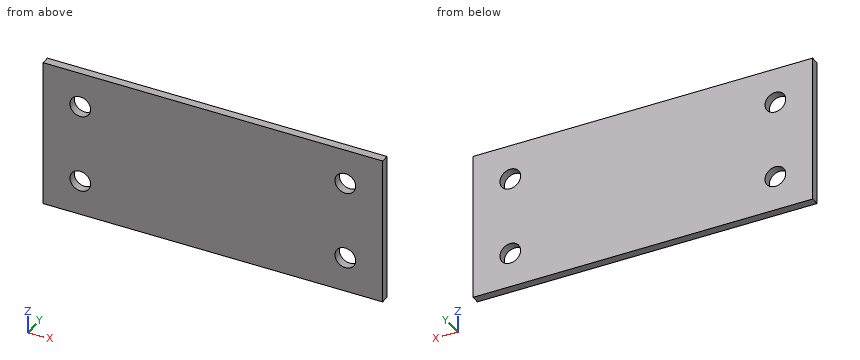
Autodesk Inventor part; units mm, degrees
ref_plane "YZ Plane" through (0, 0, 0) normal (1, 0, 0) x (0, 1, 0)
ref_plane "XZ Plane" through (0, 0, 0) normal (0, 1, 0) x (-1, 0, 0)
ref_plane "XY Plane" through (0, 0, 0) normal (0, 0, 1) x (1, 0, 0)
sketch "Sketch1" plane through (0, 0, 0) normal (0, 1, 0) x (-1, 0, 0)
  line L0 (0, -40.005) -> (0, 40.005)
  line L1 (91.1225, 0) -> (-91.1225, 0)
  line L2 (65.0875, -28.575) -> (-65.0875, -28.575)
  line L3 (-65.0875, -28.575) -> (-65.0875, 28.575)
  line L4 (-65.0875, 28.575) -> (65.0875, 28.575)
  line L5 (65.0875, 28.575) -> (65.0875, -28.575)
  circle A0 centre (50.8, -15.0812) radius 3.9688
  circle A1 centre (50.8, 15.0812) radius 3.9688
  circle A2 centre (-50.8, -15.0812) radius 3.9688
  circle A3 centre (-50.8, 15.0812) radius 3.9688
  point P0 (0, 0)
  dimension "d0" = 130.175
  dimension "d1" = 57.15
  dimension "d2" = 50.8
  dimension "d3" = 15.0813
  dimension "d4" = 7.9375
extrude "Extrusion1" add sketch "Sketch1" along normal blind 3.175
properties part number "Static_Caster_Plate"
Read the model definition and answer for the solid it produces. Units are mm, in the model's axes. Coordinates: 2 decimals unless noted, no trailing zeros. Order: outer loops, then holes, each group sorted by start corner. A loop starts at its lowest first (then second) coordinate and runs counter-clockwise, first axis right, second up. Notation, with made-up numbers: (-37.5, 70.25) - (-3.5, 70.25) arc R33 ccw to (-3.5, 104.25) - close; hole circle Ø5 at (51, 59.5). An arc over 180 degrees is marked (long way). Use one line per item in the form item = value.
(1) Section B-B, the plane y = 1.7 is taken. Give the vertices of the cut face in (x, z) (1 decimal), then the cut area to 3 significant figures.
Computed values:
outline = (-65.1, -28.6) - (65.1, -28.6) - (65.1, 28.6) - (-65.1, 28.6) - close; hole circle Ø7.9 at (-50.8, -15.1); hole circle Ø7.9 at (-50.8, 15.1); hole circle Ø7.9 at (50.8, -15.1); hole circle Ø7.9 at (50.8, 15.1)
area = 7,240 mm²
(2) Section C-C, the plane z = -17.5 is taken. Give the vertices of the cut face in (x, y) (1 decimal).
Computed values:
outline = (-65.1, 0) - (-53.9, 0) - (-53.9, 3.2) - (-65.1, 3.2) - close; (-47.7, 0) - (47.7, 0) - (47.7, 3.2) - (-47.7, 3.2) - close; (53.9, 0) - (65.1, 0) - (65.1, 3.2) - (53.9, 3.2) - close
(3) Given pin 1 Ø6.5 at (x, z) = (-50.8, -15.08) entering from -Y, flat-ended and moving along its own axis, determine where the tip first touches the part or whether it passes through.
Computed values:
pin_1 = through
(4) Section A-A, the plane x = 50.8 is taken. Give the vertices of the cut face in (y, z) (3 decimals).
Computed values:
outline = (0, -28.575) - (3.175, -28.575) - (3.175, -19.05) - (0, -19.05) - close; (0, -11.112) - (3.175, -11.112) - (3.175, 11.112) - (0, 11.112) - close; (0, 19.05) - (3.175, 19.05) - (3.175, 28.575) - (0, 28.575) - close
(5) Straight lines are drawn through the part: L1, parallel to Z at x = -50.8, y = 1.75 (3 decimals); L2, parallel to Z at x = 52.5, y = 1.3 (3 decimals); L3, parallel to X at y = 3.05, z = -17. For each, find the intervals that lie inside material, in ascending order.
Computed values:
L1 = -28.575 to -19.05, -11.112 to 11.112, 19.05 to 28.575
L2 = -28.575 to -18.667, -11.495 to 11.495, 18.667 to 28.575
L3 = -65.09 to -54.27, -47.33 to 47.33, 54.27 to 65.09
